For this review, take the finished solid that the model builds, in its own axes (mm). Face numbers are marked on the shaded views. A direction names the side the tool comes from. Round coordinates to 2 decimals unless told otherwise and drop trailing zeros. Write each loop counter-clockwise with the first axis right and the second up, starting at its lowest first coordinate (ties: lowest second). Pieces come first, ordered by that corner, then holes. Notation, with made-up numbers: (83.5, 34) - (125.5, 34) arc R8 ccw to (125.5, 43) - close; hole circle Ø7 at (-3.5, -10.75). An arc over 180 degrees is marked (long way). One line per item, written item: value. Start each with the question number.
Q1. For probe 1 along Z at (x, y) = (0, -1); probe 2 along Y at (x, z) = (2, 3.25), list the stretches that pass through material, from the lowest coordinate up.
Q2. Add section C-C on y = -1.5. Write out the cut boundary in (x, z).
Q3. Clearance check with flat-ended pins moving along their axes: pin 1 Ø2 at (x, y) = (0.5, 0.5) entering from +Z; pin 2 Ø1.2 at (y, z) = (0, 2.5) entering from -X. State where each tip first meets the part, or that it passes through.
Q4. Add section A-A on x = 0. Write out the cut boundary in (y, z).
Q5. Tool access review of the marked faces 3 and 4: name each direction out of +Z, -Z, +X, -X, +Y, -Y from which nothing blocks a thin tool from reaching the whole face with its end or side.
Q6. Add section D-D on x = 1.5. Give the number of separate pieces and of enclosed holes in the cut face, and give its area (3 significant figures).
Q7. Mouldability with a two-part tool opening along Y and no side actions: class the marked faces 1 and 2 as +Y half, -Y half, draft (parallel to the pull), parting line (faces both ways), or undercut.
Q8. Add section B-B on y = 1.6. Write out the cut boundary in (x, z).
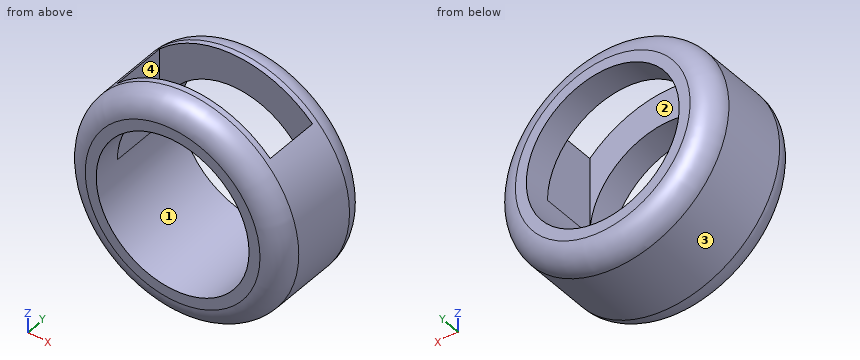
Autodesk Fusion 360 part; units mm, degrees
sketch "Sketch1" plane through (0, 0, 0) normal (0, 1, 0) x (1, 0, 0)
  circle A0 centre (0, 0) radius 3.5
  circle A1 centre (0, 0) radius 5
  dimension "d1" = 7
  dimension "d2" = 10
extrude "Extrude1" add sketch "Sketch1" along normal blind 3 and the other way blind 2
sketch "Sketch2" plane through (0, 0, 0) normal (0, 0, 1) x (1, 0, 0)
  line L0 (3.5, -0.75) -> (-3.5, -0.75)
  line L1 (-3.5, -0.75) -> (-3.5, 1.75)
  line L2 (-3.5, 1.75) -> (3.5, 1.75)
  line L3 (3.5, 1.75) -> (3.5, -0.75)
  line L4 (0, 0) -> (-3.5, 0)
  line L5 (0, 0) -> (0, 1.75)
  dimension "d7" = 7
  dimension "d8" = 2.5
  dimension "d15" = 3.5
  dimension "d16" = 1.75
extrude "Extrude2" cut sketch "Sketch2" along normal blind 5
fillet "Fillet1" radius 1 1 edges at (-4.6616, 3, 1.8081)
fillet "Fillet2" radius 1 1 edges at (-4.6616, -2, -1.8081)
Result set:
1. probe 1: z = -5 to -3.5, 3.5 to 5
1. probe 2: y = -2 to -0.75, 1.75 to 3
2. outline: circle Ø9.73 at (0, 0); hole circle Ø7 at (0, 0)
3. pin 1: stops at z = -3.16
3. pin 2: stops at x = -4.62
4. outline: (-2, -4) arc R1 ccw to (-1, -5) - (2, -5) arc R1 ccw to (3, -4) - (3, -3.5) - (-2, -3.5) - close; (-2, 3.5) - (-0.75, 3.5) - (-0.75, 5) - (-1, 5) arc R1 ccw to (-2, 4) - close; (1.75, 3.5) - (3, 3.5) - (3, 4) arc R1 ccw to (2, 5) - (1.75, 5) - close
5. face 3: +Y, -Y
5. face 4: +Z
6. separate pieces: 3
6. enclosed holes: 0
6. area: 11.2 mm^2
7. face 1: draft
7. face 2: undercut
8. outline: (-3.5, 0) - (-3.5, 3.57) arc R5 ccw (long way) to (3.5, 3.57) - (3.5, 0) arc R3.5 cw to start
